Solid Edge part; units mm, degrees
sketch "Sketch1" plane through (0, 0, 0) normal (0, 0, 1) x (1, 0, 0)
  circle A0 centre (0, 0) radius 11
  circle A1 centre (0, 0) radius 4
extrude "Protrusion1" add sketch "Sketch1" along normal mid plane 7
sketch "Sketch2" plane through (0, 0, 0) normal (0, -1, 0) x (1, 0, 0)
  line L0 (-6, -3.5) -> (-6, -2.5)
  line L1 (-6, -2.5) -> (-9, -2.5)
  line L2 (-9, -2.5) -> (-9, -3.5)
  dimension "D1" = 6
revolve "RevolvedCutout1" cut sketch "Sketch2" angle 360 about axis through (0, 0, 54) along (0, 0, -1) material side at (-6.05, 0, -3)
mirror "Mirror1" about plane through (0, 0, 0) normal (0, 0, 1) of "RevolvedCutout1"
properties material "Stainless steel"
Check sheet for the modelled part. Datum: model origin and axes. Units: mm. A direction names the side the tool comes from. Coordinates: 2 decimals unless noted, no trailing zeros. Write each loop counter-clockwise with the first axis right and the second up, starting at its lowest first coordinate (ties: lowest second). Pieces come first, ordered by that corner, then holes. Notation, with made-up numbers: M -37,17.5 L -6,17.5 A18 ccw -6,30.5 Z; hole C 28,33 d7. An arc over 180 degrees is marked long. Use one line per item in the form item = value.
Item 1: Gauge pin test, flat ends, axial feed: pin 1 Ø3 at (y, z) = (-8, 1.5) entering from +X; pin 2 Ø1.5 at (x, z) = (6.5, 2.5) entering from +Y; pin 3 Ø2 at (y, z) = (-6, 1.5) entering from -X. Record the tip position at first contact, or that the pin passes through.
Answer below:
pin_1 = 8.87
pin_2 = 9.38
pin_3 = -9.8
Item 2: Material ranges on L1, parallel to Y at x = 0, z = 2.9; L2, parallel to Y at x = 2.5, z = 3.25; L3, parallel to Y at x = -4.5, z = -2.75, recorded low to high. Write a range as from..to.
Answer below:
L1 = -11..-9, -6..-4, 4..6, 9..11
L2 = -10.71..-8.65, -5.45..-3.12, 3.12..5.45, 8.65..10.71
L3 = -10.04..-7.79, -3.97..3.97, 7.79..10.04
Item 3: Set-up check for faces 4 (the face through (-2, -6, -2.5)), 5 (the face through (2, -9, -3.5)), 6 (the face through (2, -6, 2.5)): record each of +Z, -Z, +X, -X, +Y, -Y from which the full face is reachable in a straight line by a thin tool's end or side.
Answer below:
face_4 = -Z
face_5 = -Z, +X, -X, +Y, -Y
face_6 = +Z
Item 4: Sectioned sample at D-D, the plane x = 8. Record the cut outline in (y, z), and give its area (3 significant figures).
Answer below:
outline = M -7.55,-3.5 L -4.12,-3.5 L -4.12,-2.5 L 4.12,-2.5 L 4.12,-3.5 L 7.55,-3.5 L 7.55,3.5 L 4.12,3.5 L 4.12,2.5 L -4.12,2.5 L -4.12,3.5 L -7.55,3.5 Z
area = 89.2 mm^2
Item 5: Release check for a two-part mould opening along X. For faces 1 (the face through (2, -9, 3.5)), 2 (the face through (-2.38, 10.74, -0.05)), 3 (the face through (6, 0, 3)) record: pulls with the +X half, pulls with the -X half, needs draft (parallel to the pull), parting line crosses it, or undercut.
Answer below:
face_1 = needs draft
face_2 = parting line crosses it
face_3 = undercut
Item 6: Sectioned sample at A-A, the plane y = 0. Record the cut outline in (x, z), and give its area (3 significant figures).
Answer below:
outline = M -11,-3.5 L -9,-3.5 L -9,-2.5 L -6,-2.5 L -6,-3.5 L -4,-3.5 L -4,3.5 L -6,3.5 L -6,2.5 L -9,2.5 L -9,3.5 L -11,3.5 Z; M 4,-3.5 L 6,-3.5 L 6,-2.5 L 9,-2.5 L 9,-3.5 L 11,-3.5 L 11,3.5 L 9,3.5 L 9,2.5 L 6,2.5 L 6,3.5 L 4,3.5 Z
area = 86.0 mm^2
Item 7: Sectioned sample at C-C, the plane z = -1.25. Record the cut outline in (x, y).
Answer below:
outline = C 0,0 d22; hole C 0,0 d8
